For this review, take the finished solid that the model builds, in its own axes (mm). Face numbers are marked on the shaded views. A direction names the side the tool comes from. Coordinates: 2 decimals unless noted, no trailing zeros. Loops run counter-clockwise (first coordinate to the right, second up) from the corner with the lowest first, then second, coordinate; pieces in that order, holes last. Notation, with made-up numbers: M -21.75,7.25 L 23.25,7.25 A28 cw 23.25,33.25 Z; hole C 17,-28 d6. An arc over 180 degrees is marked long. Put each result on its own line as item: value.
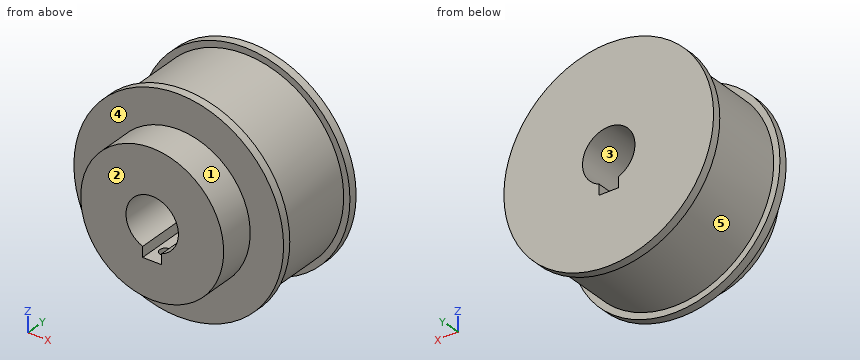
```python
from build123d import *

# Parameters (mm, degrees)
SKETCH2_R          = 5.5
CUT_EXTRUDE1_DEPTH = 33
CUT_EXTRUDE2_DEPTH = 33
SKETCH4_R          = 1.2
CUT_EXTRUDE3_DEPTH = 80


with BuildPart() as part:
    # Sketch1 → Revolve1 (revolve)
    with BuildSketch(Plane.XY, mode=Mode.PRIVATE) as revolve1_sk:
        Polygon((4, 0), (15, 0), (15, 7.5), (22, 7.5), (22, 9.25), (20.69, 9.25), (20.69, 26.25), (22, 26.25), (22, 28), (4, 28), align=None)
    revolve(revolve1_sk.sketch.rotate(Axis((0, 0, 0), (0, 1, 0)), 90), axis=Axis((0, 0, 0), (0, 1, 0)))

    # Sketch2 → Cut-Extrude1 (cut)
    with BuildSketch(Plane(origin=(0, 28, 0), x_dir=(1, 0, 0), z_dir=(0, 1, 0))):
        with Locations(Location((0, 0, 0), (0, 0, 270))):
            Circle(SKETCH2_R)
    extrude(amount=-CUT_EXTRUDE1_DEPTH, mode=Mode.SUBTRACT)

    # Sketch3 → Cut-Extrude2 (cut)
    with BuildSketch(Plane(origin=(0, 28, 0), x_dir=(1, 0, 0), z_dir=(0, 1, 0))):
        with BuildLine():
            Line((-2, 7.3), (-2, 5.123475383))
            ThreePointArc((-2, 5.123475383), (0, 5.5), (2, 5.123475383))
            Line((2, 5.123475383), (2, 7.3))
            Line((2, 7.3), (-2, 7.3))
        make_face()
    extrude(amount=-CUT_EXTRUDE2_DEPTH, mode=Mode.SUBTRACT)

    # Sketch4 → Cut-Extrude3 (cut)
    with BuildSketch(Plane.XY.offset(-7.3)):
        with Locations((0, 3.75)):
            Circle(SKETCH4_R)
    extrude(amount=-CUT_EXTRUDE3_DEPTH, mode=Mode.SUBTRACT)


solid = part.part
```
(1) Tool access review of the marked faces 1 and 2: name each direction out of +Z, -Z, +X, -X, +Y, -Y from which nothing blocks a thin tool from reaching the whole face with its end or side.
Determined:
face 1: -Y
face 2: +Z, -Z, +X, -X, -Y
(2) Wall thickness on line 1 along X through (y, z) = (18, 0); line 2 along Y through (x, z) = (0, -10); line 3 along Y through (x, z) = (9.5, 15.5): over which ranges is each line inside the solid? List them lowest first. Write a range as [from, to].
Determined:
line 1: x = [-20.69, -5.5], [5.5, 20.69]
line 2: y = [0, 2.55], [4.95, 28]
line 3: y = [7.5, 28]
(3) Add section D-D (x = -18). Write out the cut boundary in (y, z).
Determined:
outline: M 7.5,-12.65 L 9.25,-12.65 L 9.25,-10.2 L 26.25,-10.2 L 26.25,-12.65 L 28,-12.65 L 28,12.65 L 26.25,12.65 L 26.25,10.2 L 9.25,10.2 L 9.25,12.65 L 7.5,12.65 Z
(4) Draft analysis for pull direction X (two halves, no side actions). For the marked faces 3, 4 and 5, state which applies: +X half, -X half, draft (parallel to the pull), parting line (faces both ways), or undercut.
Determined:
face 3: undercut
face 4: draft
face 5: parting line
(5) For pin 1 (10 mm diameter, centred on y = 18, z = 5, fed in from -X); pin 2 (3 mm diameter, centred on x = -0.5, y = 20, fed in from +Z); pin 3 (1.7 mm diameter, centred on y = 17.5, z = -6, fed in from -X), all flat-tipped, find the tip position at first contact; note any pin that passes through.
Determined:
pin 1: stops at x = -20.69
pin 2: stops at z = 20.69
pin 3: stops at x = -20.04
(6) Add section C-C (y = 13.75). Write out the cut boundary in (x, z).
Determined:
outline: C 0,0 d41.38; hole M -2,-7.3 L 2,-7.3 L 2,-5.12 A5.5 ccw long -2,-5.12 Z
(7) Add section B-B (z = 0). Write out the cut boundary in (x, y).
Determined:
outline: M -22,7.5 L -15,7.5 L -15,0 L -5.5,0 L -5.5,28 L -22,28 L -22,26.25 L -20.69,26.25 L -20.69,9.25 L -22,9.25 Z; M 5.5,0 L 15,0 L 15,7.5 L 22,7.5 L 22,9.25 L 20.69,9.25 L 20.69,26.25 L 22,26.25 L 22,28 L 5.5,28 Z
(8) Add section A-A (x = 0). Write out the cut boundary in (y, z).
Determined:
outline: M 0,-15 L 2.55,-15 L 2.55,-7.3 L 0,-7.3 Z; M 0,5.5 L 28,5.5 L 28,22 L 26.25,22 L 26.25,20.69 L 9.25,20.69 L 9.25,22 L 7.5,22 L 7.5,15 L 0,15 Z; M 4.95,-15 L 7.5,-15 L 7.5,-22 L 9.25,-22 L 9.25,-20.69 L 26.25,-20.69 L 26.25,-22 L 28,-22 L 28,-7.3 L 4.95,-7.3 Z
